The model under review builds one solid part; all positions refer to its coordinate system, in mm. Face numbers are marked on the shaded views. A direction names the side the tool comes from. Round coordinates to 2 decimals unless told otherwise and drop trailing zeros. Write each loop counter-clockwise with the first axis right and the second up, starting at its lowest first coordinate (ties: lowest second). Pieces come first, ordered by that corner, then holes. Notation, with made-up numbers: (52.5, 60) - (72.5, 60) arc R23 cw to (72.5, 79) - close; hole circle Ø10 at (65, 11.25). An arc over 180 degrees is marked (long way). One line per question, with ' | ' between items. Start each with the question number.
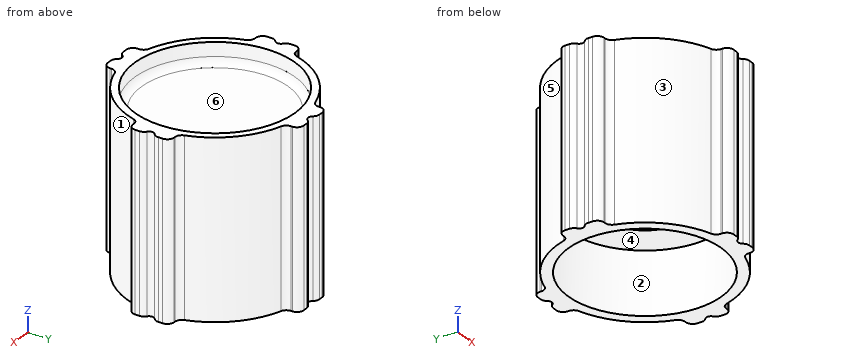
```python
from build123d import *

# Parameters (mm, degrees)
SKETCH1_R           = 6.35
BOSS_EXTRUDE1_DEPTH = 12.7
SKETCH2_W           = 14.3
SKETCH2_H           = 3
BOSS_EXTRUDE2_DEPTH = 12.7
SKETCH3_W           = 3
SKETCH3_H           = 14.3
BOSS_EXTRUDE3_DEPTH = 12.7
SKETCH4_R           = 0.35
CUT_EXTRUDE2_DEPTH  = 12.7
FILLET1_R           = 0.5
FILLET2_R           = 0.5
CUT_EXTRUDE3_START  = 12.7
SKETCH5_R           = 5.815
CUT_EXTRUDE3_DEPTH  = 1.5
FILLET3_R           = 0.5
SKETCH7_R           = 3
CUT_EXTRUDE5_DEPTH  = 9.5
BOSS_EXTRUDE4_START = 1
SKETCH8_W           = 6
SKETCH8_H           = 1.56
BOSS_EXTRUDE4_DEPTH = 9.5
SKETCH6_R           = 5.565
CUT_EXTRUDE4_DEPTH  = 4.5


with BuildPart() as part:
    # Sketch1 → Boss-Extrude1 (new body)
    with BuildSketch(Plane.XY):
        Circle(SKETCH1_R)
    extrude(amount=BOSS_EXTRUDE1_DEPTH)

    # Sketch2 → Boss-Extrude2 (add)
    with BuildSketch(Plane.XY):
        Rectangle(SKETCH2_W, SKETCH2_H)
    extrude(amount=BOSS_EXTRUDE2_DEPTH)

    # Sketch3 → Boss-Extrude3 (add)
    with BuildSketch(Plane.XY):
        Rectangle(SKETCH3_W, SKETCH3_H)
    extrude(amount=BOSS_EXTRUDE3_DEPTH)

    # Sketch4 → Cut-Extrude2 (cut)
    with BuildSketch(Plane.XY):
        with Locations((0, 7.15)):
            Circle(SKETCH4_R)
        with Locations((7.15, 0)):
            Circle(SKETCH4_R)
        with Locations((-7.15, 0)):
            Circle(SKETCH4_R)
        with Locations((0, -7.15)):
            Circle(SKETCH4_R)
    extrude(amount=CUT_EXTRUDE2_DEPTH, mode=Mode.SUBTRACT)

    # Fillet1
    fillet1_edges = [part.edges().sort_by_distance(p)[0] for p in [
        (7.15, 1.5, 6.35),
        (-7.15, -1.5, 6.35),
        (7.15, -1.5, 6.35),
        (-7.15, 1.5, 6.35),
        (1.5, -7.15, 6.35),
        (-1.5, 7.15, 6.35),
        (1.5, 7.15, 6.35),
        (-1.5, -7.15, 6.35),
    ]]
    fillet(fillet1_edges, radius=FILLET1_R)

    # Fillet2
    fillet2_edges = [part.edges().sort_by_distance(p)[0] for p in [
        (-6.170291727, 1.5, 6.35),
        (6.170291727, 1.5, 6.35),
        (6.170291727, -1.5, 6.35),
        (-6.170291727, -1.5, 6.35),
        (1.5, 6.170291727, 6.35),
        (1.5, -6.170291727, 6.35),
        (-1.5, 6.170291727, 6.35),
        (-1.5, -6.170291727, 6.35),
        (0.35, 7.15, 6.35),
        (-0.35, 7.15, 6.35),
        (-0.35, -7.15, 6.35),
        (0.35, -7.15, 6.35),
        (7.15, -0.35, 6.35),
        (7.15, 0.35, 6.35),
        (-7.15, 0.35, 6.35),
        (-7.15, -0.35, 6.35),
    ]]
    fillet(fillet2_edges, radius=FILLET2_R)

    # Sketch5 → Cut-Extrude3 (cut)
    with BuildSketch(Plane.XY.offset(CUT_EXTRUDE3_START)):
        Circle(SKETCH5_R)
    extrude(amount=-CUT_EXTRUDE3_DEPTH, mode=Mode.SUBTRACT)

    # Fillet3
    fillet3_edges = [part.edges().sort_by_distance(p)[0] for p in [
        (-5.815, 0, 11.2),
    ]]
    fillet(fillet3_edges, radius=FILLET3_R)

    # Sketch7 → Cut-Extrude5 (cut)
    with BuildSketch(Plane.XY):
        Circle(SKETCH7_R)
    extrude(amount=CUT_EXTRUDE5_DEPTH, mode=Mode.SUBTRACT)

    # Sketch8 → Boss-Extrude4 (add)
    with BuildSketch(Plane.XY.offset(BOSS_EXTRUDE4_START)):
        with Locations((0, -2.22)):
            Rectangle(SKETCH8_W, SKETCH8_H)
    extrude(amount=BOSS_EXTRUDE4_DEPTH)

    # Sketch6 → Cut-Extrude4 (cut)
    with BuildSketch(Plane.XY):
        Circle(SKETCH6_R)
    extrude(amount=CUT_EXTRUDE4_DEPTH, mode=Mode.SUBTRACT)


solid = part.part
```
1. Add section A-A, the plane y = 0. Write out the cut boundary in (x, z) (3 decimals), then the cut area to 3 significant figures.
2. Add section B-B, the plane x = 0. Write out the cut boundary in (y, z) (3 decimals), then the cut area to 3 significant figures.
3. The part is to be moulded in two halves that separate along Y. For the marked faces 3, 4, 5 and 6, say which applies: pulls with the +Y half, pulls with the -Y half, needs draft (parallel to the pull), parting line crosses it, or undercut.
4. Clearance check with flat-ended pins moving along their axes: P1, Ø1.5, axis at x = -1.5, z = 4.5, coming from the +Y side; P2, Ø1, axis at x = 5.5, z = 7.5, coming from the +Y side; P3, Ø5, axis at y = 4.5, z = 3.5, coming from the +X side; P4, Ø5.5, axis at x = -1, y = -1, coming from the +Z side. State where each tip first meets the part, or that it passes through.
5. Machinability: for the marked faces 1 and 2, which of the approach directions +Z, -Z, +X, -X, +Y, -Y give a long, thin tool a straight path to every point of the face, cutting with its end or side? Answer none if there is none.
6. Wall thickness on line 1 along Y through (x, z) = (0, 8.35); line 2 along Y through (x, z) = (0, 2.35) (3 decimals); line 3 along X through (y, z) = (0, 8): over which ranges is each line inside the solid? List them lowest first. Write a range as [from, to].
Geometry check:
1) outline: (-6.8, 0) - (-5.565, 0) - (-5.565, 4.5) - (-3, 4.5) - (-3, 9.5) - (3, 9.5) - (3, 4.5) - (5.565, 4.5) - (5.565, 0) - (6.8, 0) - (6.8, 12.7) - (5.815, 12.7) - (5.815, 11.7) arc R0.5 cw to (5.315, 11.2) - (-5.315, 11.2) arc R0.5 cw to (-5.815, 11.7) - (-5.815, 12.7) - (-6.8, 12.7) - close | area: 75.3 mm2
2) outline: (-6.8, 0) - (-5.565, 0) - (-5.565, 4.5) - (-1.44, 4.5) - (-1.44, 9.5) - (3, 9.5) - (3, 4.5) - (5.565, 4.5) - (5.565, 0) - (6.8, 0) - (6.8, 12.7) - (5.815, 12.7) - (5.815, 11.7) arc R0.5 cw to (5.315, 11.2) - (-5.315, 11.2) arc R0.5 cw to (-5.815, 11.7) - (-5.815, 12.7) - (-6.8, 12.7) - close | area: 83.1 mm2
3) face 3: pulls with the -Y half | face 4: undercut | face 5: pulls with the +Y half | face 6: undercut
4) P1: stops at y = 7.15 | P2: stops at y = 3.91 | P3: stops at x = 6.03 | P4: stops at z = 11.2
5) face 1: +Z, -Z, +X, -Y | face 2: -Z
6) line 1: y = [-6.8, -1.44], [3, 6.8] | line 2: y = [-6.8, -5.565], [5.565, 6.8] | line 3: x = [-6.8, -3], [3, 6.8]
